```python
from build123d import *

# Parameters (mm, degrees)
F0_W      = 3
F0_H      = 8
F1_DEPTH  = 3
F2_DEPTH  = 4.9
F3_DEPTH  = 4.9
F5_DEPTH  = 3
F7_DEPTH  = 3
F8_DEPTH  = 25
F9_DEPTH  = 1
F11_DEPTH = 3
F12_R     = 1.8630386708
F13_DEPTH = 1
F14_R     = 1.9023250727
F15_DEPTH = 1
F16_R     = 1.25
F17_DEPTH = 2
F18_DEPTH = 1


with BuildPart() as f1:
    # F0 (on Top) → F1 (new body)
    with BuildSketch(Plane.XY):
        with BuildLine():
            Line((9.35, -30.6), (9.35, 0))
            ThreePointArc((9.35, 0), (0, -9.35), (-9.35, 0))
            Line((-9.35, 0), (-9.35, -30.6))
            Line((-9.35, -30.6), (9.35, -30.6))
        make_face()
        with Locations((-4.25, -20.6)):
            Rectangle(F0_W, F0_H, mode=Mode.SUBTRACT)
        with Locations((4.25, -20.6)):
            Rectangle(F0_W, F0_H, mode=Mode.SUBTRACT)
        with BuildLine():
            ThreePointArc((-9.35, 0), (0, -9.35), (9.35, 0))
            ThreePointArc((9.35, 0), (0, 9.35), (-9.35, 0))
        make_face()
        with Locations((4.25, -20.6)):
            Rectangle(F0_W, F0_H)
        with Locations((-4.25, -20.6)):
            Rectangle(F0_W, F0_H)
    extrude(amount=-F1_DEPTH)

    # F0 (on Top) → F2 (join)
    with BuildSketch(Plane.XY):
        with Locations((4.25, -20.6)):
            Rectangle(F0_W, F0_H)
    extrude(amount=F2_DEPTH)

    # F0 (on Top) → F3 (join)
    with BuildSketch(Plane.XY):
        with Locations((-4.25, -20.6)):
            Rectangle(F0_W, F0_H)
    extrude(amount=F3_DEPTH)

    # F4 (on face) → F5 (join)
    with BuildSketch(Plane(origin=(-5.75, 0, 0), x_dir=(0, -1, 0), z_dir=(-1, 0, 0))):
        with BuildLine():
            Line((16.6, 4.9), (24.6, 4.9))
            ThreePointArc((24.6, 4.9), (20.6, 8.9), (16.6, 4.9))
        make_face()
    extrude(amount=-F5_DEPTH)

    # F6 (on face) → F7 (join)
    with BuildSketch(Plane.YZ.offset(5.75)):
        with BuildLine():
            Line((-17.944, 4.9), (-16.6, 4.9))
            ThreePointArc((-16.6, 4.9), (-20.6, 8.9), (-24.6, 4.9))
            Line((-24.6, 4.9), (-23.256, 4.9))
            Line((-23.256, 4.9), (-21.928, 7.2001634725))
            Line((-21.928, 7.2001634725), (-19.272, 7.2001634725))
            Line((-19.272, 7.2001634725), (-17.944, 4.9))
        make_face()
        with BuildLine():
            Line((-19.311, 4.9), (-17.944, 4.9))
            Line((-17.944, 4.9), (-19.272, 7.2001634725))
            Line((-19.272, 7.2001634725), (-21.928, 7.2001634725))
            Line((-21.928, 7.2001634725), (-23.256, 4.9))
            Line((-23.256, 4.9), (-21.889, 4.9))
            ThreePointArc((-21.889, 4.9), (-20.6, 6.189), (-19.311, 4.9))
        make_face()
    extrude(amount=-F7_DEPTH)

    # F6 (on face) → F8 (cut)
    with BuildSketch(Plane.YZ.offset(5.75)):
        with BuildLine():
            Line((-21.889, 4.9), (-19.311, 4.9))
            ThreePointArc((-19.311, 4.9), (-20.6, 6.189), (-21.889, 4.9))
        make_face()
        with BuildLine():
            ThreePointArc((-21.889, 4.9), (-20.6, 3.611), (-19.311, 4.9))
            Line((-19.311, 4.9), (-21.889, 4.9))
        make_face()
    extrude(amount=-F8_DEPTH, mode=Mode.SUBTRACT)

    # F6 (on face) → F9 (cut)
    with BuildSketch(Plane.YZ.offset(5.75)):
        with BuildLine():
            Line((-19.311, 4.9), (-17.944, 4.9))
            Line((-17.944, 4.9), (-19.272, 7.2001634725))
            Line((-19.272, 7.2001634725), (-21.928, 7.2001634725))
            Line((-21.928, 7.2001634725), (-23.256, 4.9))
            Line((-23.256, 4.9), (-21.889, 4.9))
            ThreePointArc((-21.889, 4.9), (-20.6, 6.189), (-19.311, 4.9))
        make_face()
        with BuildLine():
            Line((-19.272, 2.5998365275), (-17.944, 4.9))
            Line((-17.944, 4.9), (-19.311, 4.9))
            ThreePointArc((-19.311, 4.9), (-20.6, 3.611), (-21.889, 4.9))
            Line((-21.889, 4.9), (-23.256, 4.9))
            Line((-23.256, 4.9), (-21.928, 2.5998365275))
            Line((-21.928, 2.5998365275), (-19.272, 2.5998365275))
        make_face()
    extrude(amount=-F9_DEPTH, mode=Mode.SUBTRACT)

    # F10 (on face) → F11 (join)
    with BuildSketch(Plane.XY):
        with BuildLine():
            Line((9.85, -31.1), (9.85, 0))
            ThreePointArc((9.85, 0), (0, 9.85), (-9.85, 0))
            Line((-9.85, 0), (-9.85, -31.1))
            Line((-9.85, -31.1), (9.85, -31.1))
        make_face()
        with BuildLine():
            Line((-9.35, -30.6), (-9.35, 0))
            ThreePointArc((-9.35, 0), (0, 9.35), (9.35, 0))
            Line((9.35, 0), (9.35, -30.6))
            Line((9.35, -30.6), (-9.35, -30.6))
        make_face(mode=Mode.SUBTRACT)
    extrude(amount=-F11_DEPTH)

    # F12 (on face) → F13 (join)
    with BuildSketch(Plane.YZ.offset(-2.75)):
        with Locations((-20.6, 4.9)):
            Circle(F12_R)
    extrude(amount=-F13_DEPTH)

    # F14 (on face) → F15 (join)
    with BuildSketch(Plane(origin=(2.75, 0, 0), x_dir=(0, -1, 0), z_dir=(-1, 0, 0))):
        with Locations((20.6, 4.9)):
            Circle(F14_R)
    extrude(amount=-F15_DEPTH)

    # F16 (on face) → F17 (join)
    with BuildSketch(Plane.XY):
        with Locations((6.65, -3.1)):
            Circle(F16_R)
    extrude(amount=F17_DEPTH)

    # F18 (add): a face of the model
    f18_faces = [f1.faces().sort_by_distance(p)[0] for p in [
        (-3.75, -20.6, 4.9),
    ]]
    extrude(f18_faces, amount=F18_DEPTH)


solid = f1.part
```
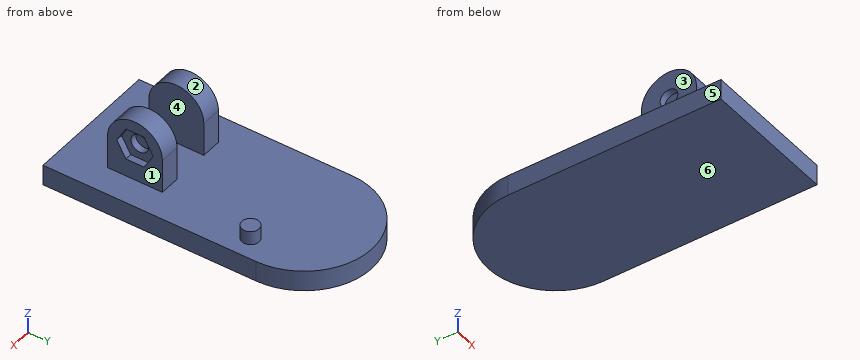
Can you work these out from the model? Positions are in its coordinate system, mm. Face numbers are marked on the shaded views. A direction names the side the tool comes from. Coordinates: 2 decimals unless noted, no trailing zeros. Loops run counter-clockwise (first coordinate to the right, second up) from the corner with the lowest first, then second, coordinate; pieces in that order, holes last.
Item 1: I'm going to push flat-ended pins straight in: pin 1 (2.5 mm diameter, centred on x = -3.5, z = 3.5, fed in from +Y); pin 2 (5 mm diameter, centred on y = -21, z = 4, fed in from +X); pin 3 (6.5 mm diameter, centred on y = -20.5, z = 5, fed in from -X). Where does each tip first touch, or does it pass through?
Answers below:
pin 1: stops at y = -16.6
pin 2: stops at x = 5.75
pin 3: stops at x = -5.75
Item 2: Suppose I cut it at D-D (x = 0). Please give me the cut outline in (y, z).
Answers below:
outline: (-31.1, -3) - (9.85, -3) - (9.85, 0) - (-31.1, 0) - close
Item 3: Which directions (+Z, -Z, +X, -X, +Y, -Y) give clear straight access to the entire face, cutting with the end or side of a thin tool? Please do the marked faces 1, 2 and 3.
Answers below:
face 1: +Z, +X, -Y
face 2: +Z, +X, -X
face 3: +Z, -X, +Y, -Y
Item 4: Suppose I cut it at A-A (y = -3.1). Please give me the cut outline in (x, z), then the cut area to 3 significant figures.
Answers below:
outline: (-9.85, -3) - (9.85, -3) - (9.85, 0) - (7.9, 0) - (7.9, 2) - (5.4, 2) - (5.4, 0) - (-9.85, 0) - close
area: 64.1 mm2
Item 5: Suppose I cut it at B-B (x = 4.25). Please give me the cut outline in (y, z), then the cut area to 3 significant figures.
Answers below:
outline: (-31.1, -3) - (8.89, -3) - (8.89, 0) - (-16.6, 0) - (-16.6, 4.9) arc R4 ccw to (-24.6, 4.9) - (-24.6, 0) - (-31.1, 0) - close; hole circle Ø2.58 at (-20.6, 4.9)
area: 179 mm2
Item 6: Please list where these lines run through material, in increasing order: L1, parallel to X at y = -21, z = 7.75; L2, parallel to Y at x = -5.1, z = 4.9; L3, parallel to Z at x = 4.15, y = -20.6.
Answers below:
L1: x = -5.75 to -2.75, 2.75 to 5.75
L2: y = -24.6 to -21.89, -19.31 to -16.6
L3: z = -3 to 3.61, 6.19 to 8.9
Item 7: Suppose I cut it at C-C (z = 5.5). Please give me the cut outline in (x, y), then the cut area to 3 significant figures.
Answers below:
outline: (-5.75, -24.55) - (-2.75, -24.55) - (-2.75, -16.65) - (-5.75, -16.65) - (-5.75, -19.46) - (-4.75, -19.46) - (-4.75, -21.74) - (-5.75, -21.74) - close; (2.75, -24.55) - (5.75, -24.55) - (5.75, -22.91) - (4.75, -22.91) - (4.75, -21.74) - (3.75, -21.74) - (3.75, -19.46) - (4.75, -19.46) - (4.75, -18.29) - (5.75, -18.29) - (5.75, -16.65) - (2.75, -16.65) - close
area: 38.3 mm2
Item 8: If we mould it in two halves opening along X, with no side actions, what happens to the marked faces 4, 5 and 6? For each: released by +X, released by -X, zero draft, split by the parting line, or undercut.
Answers below:
face 4: undercut
face 5: released by -X
face 6: zero draft
